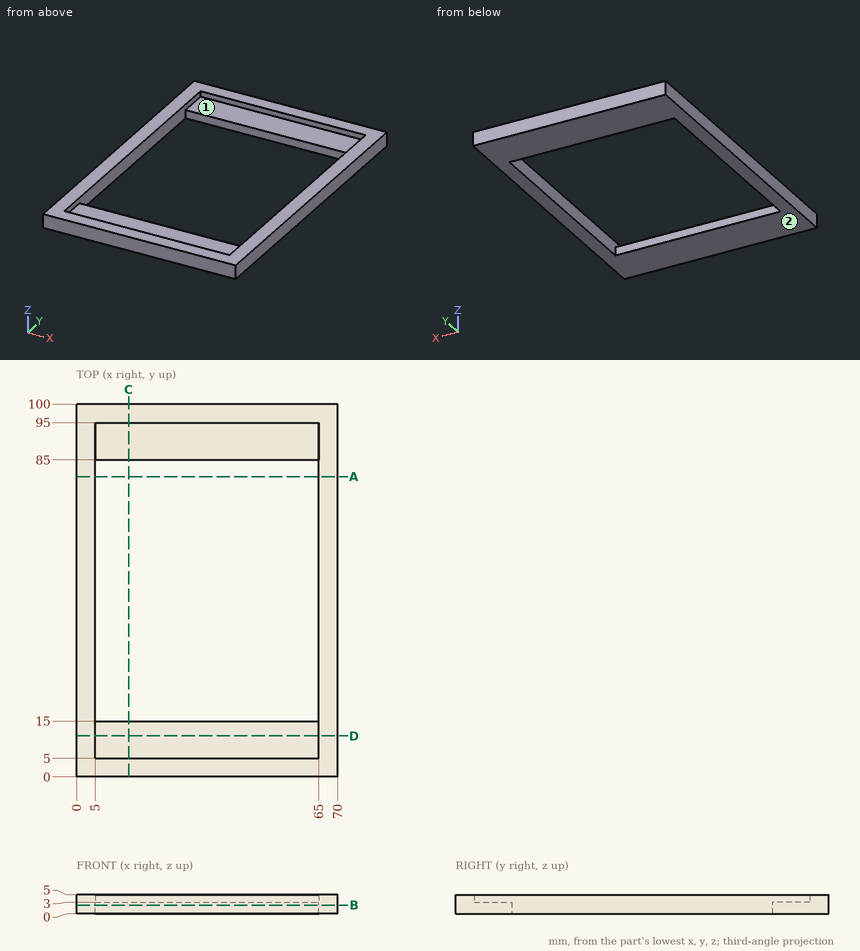
Geometry check sheet. Reference: drawing and pictorial views, mm from the part's lowest x, y, z. Coordinates: 2 decimals unless noted, no trailing zeros. Loops run counter-clockwise (first coordinate to the right, second up) from the corner with the lowest first, then second, coordinate; pieces in that order, holes last. Notation, with made-up numbers: (-31.75, 57.5) -> (8.25, 57.5) arc R24 ccw to (8.25, 68.5) -> close; hole circle Ø1 at (9, -36). An arc over 180 degrees is marked (long way). Write item = value, one per line. Start each with the question number.
1. Section check D-D on y = 11. Record the cut outline in (x, z), then the cut area to 3 significant figures.
2. Section check C-C on x = 14. Record the cut outline in (y, z), then the cut area to 3 significant figures.
3. Section check B-B on z = 2.25. Record the cut outline in (x, y), then the cut area to 3 significant figures.
4. Draft check along X on the marked faces 1 and 2. Enter one of: released by +X, released by -X, zero draft, split by the parting line, or undercut.
5. Material ranges on line 1 (Y direction, x = 12.5, z = 0.5); line 2 (X direction, y = 16, z = 3.75); line 3 (Y direction, x = 61, z = 3.65), recorded low to high.
6. Depth check by flat-ended pin: P1, Ø8, axis at x = 27.5, y = 10, coming from the +Z side. Enter the tip coordinate at first touch or a pass-through.
7. Section check A-A on y = 80.5. Record the cut outline in (x, z).
Responses:
q1.outline = (0, 0) -> (70, 0) -> (70, 5) -> (65, 5) -> (65, 3) -> (5, 3) -> (5, 5) -> (0, 5) -> close
q1.area = 230 mm2
q2.outline = (0, 0) -> (15, 0) -> (15, 3) -> (5, 3) -> (5, 5) -> (0, 5) -> close; (85, 0) -> (100, 0) -> (100, 5) -> (95, 5) -> (95, 3) -> (85, 3) -> close
q2.area = 110 mm2
q3.outline = (0, 0) -> (70, 0) -> (70, 100) -> (0, 100) -> close; hole (5, 15) -> (65, 15) -> (65, 85) -> (5, 85) -> close
q3.area = 2,800 mm2
q4.face_1 = undercut
q4.face_2 = zero draft
q5.line_1 = 0 to 15, 85 to 100
q5.line_2 = 0 to 5, 65 to 70
q5.line_3 = 0 to 5, 95 to 100
q6.P1 = 3
q7.outline = (0, 0) -> (5, 0) -> (5, 5) -> (0, 5) -> close; (65, 0) -> (70, 0) -> (70, 5) -> (65, 5) -> close
